from build123d import *

# Parameters (mm, degrees)
F0_W      = 127
F0_H      = 127
F1_DEPTH  = 127
F2_R      = 12.7
F3_DEPTH  = 6.35
F4_R      = 12.7
F5_DEPTH  = 6.35
F6_R      = 12.7
F7_DEPTH  = 6.35
F8_R      = 12.7
F9_DEPTH  = 6.35
F10_R     = 12.7
F11_DEPTH = 6.35
F12_R     = 12.7
F13_DEPTH = 6.35
F14_R     = 12.7
F15_DEPTH = 6.35
F16_R     = 12.7
F17_DEPTH = 6.35
F18_R     = 12.7
F19_DEPTH = 6.35
F20_R     = 12.2418661496
F21_DEPTH = 6.35
F22_R     = 12.7
F23_DEPTH = 6.35
F25_R     = 12.7
F26_DEPTH = 6.35
F27_R     = 12.7
F28_DEPTH = 6.35
F29_R     = 12.7
F30_DEPTH = 6.35
F31_R     = 12.7
F32_DEPTH = 6.35
F33_R     = 12.7
F34_DEPTH = 6.35
F35_R     = 12.7
F36_DEPTH = 6.35
F37_R     = 12.7
F38_DEPTH = 6.35
F39_R     = 12.7
F40_DEPTH = 6.35
F41_R     = 12.7
F42_DEPTH = 6.35
F43_R     = 12.7
F44_DEPTH = 6.35


# Not quite as in the source:
# - a length typed as a fraction of an inch, garbled in the dataset ("3 / 203.2 mm" for 3/8 in), is restored


with BuildPart() as f1:
    # F0 (on Right) → F1 (new body)
    with BuildSketch(Plane.YZ):
        with Locations((-2.1555427632, -5.2600353956)):
            Rectangle(F0_W, F0_H)
    extrude(amount=F1_DEPTH)

    # F2 (on face) → F3 (cut)
    with BuildSketch(Plane(origin=(0, 61.3444572368, 0), x_dir=(-1, 0, 0), z_dir=(0, 1, 0))):
        with Locations((-63.2817981055, -5.2596604964)):
            Circle(F2_R)
    extrude(amount=-F3_DEPTH, mode=Mode.SUBTRACT)

    # F4 (on face) → F5 (cut)
    with BuildSketch(Plane(origin=(0, 0, 0), x_dir=(0, -1, 0), z_dir=(-1, 0, 0))):
        with Locations((2.032, -6.35)):
            Circle(F4_R)
    extrude(amount=-F5_DEPTH, mode=Mode.SUBTRACT)

    # F6 (on face) → F7 (cut)
    with BuildSketch(Plane(origin=(0, 0, 0), x_dir=(0, -1, 0), z_dir=(-1, 0, 0))):
        with Locations((-39.1194572368, 36.0149646044)):
            Circle(F6_R)
    extrude(amount=-F7_DEPTH, mode=Mode.SUBTRACT)

    # F8 (on face) → F9 (cut)
    with BuildSketch(Plane(origin=(0, 0, 0), x_dir=(0, -1, 0), z_dir=(-1, 0, 0))):
        with Locations((43.4305427632, 36.0149646044)):
            Circle(F8_R)
    extrude(amount=-F9_DEPTH, mode=Mode.SUBTRACT)

    # F10 (on face) → F11 (cut)
    with BuildSketch(Plane(origin=(0, 0, 0), x_dir=(0, -1, 0), z_dir=(-1, 0, 0))):
        with Locations((-39.1194572368, -46.5350353956)):
            Circle(F10_R)
    extrude(amount=-F11_DEPTH, mode=Mode.SUBTRACT)

    # F12 (on face) → F13 (cut)
    with BuildSketch(Plane(origin=(0, 0, 0), x_dir=(0, -1, 0), z_dir=(-1, 0, 0))):
        with Locations((43.4305427632, -46.5350353956)):
            Circle(F12_R)
    extrude(amount=-F13_DEPTH, mode=Mode.SUBTRACT)

    # F14 (on face) → F15 (cut)
    with BuildSketch(Plane.YZ.offset(127)):
        with Locations((39.1194572368, -46.5350353956)):
            Circle(F14_R)
    extrude(amount=-F15_DEPTH, mode=Mode.SUBTRACT)

    # F16 (on face) → F17 (cut)
    with BuildSketch(Plane.YZ.offset(127)):
        with Locations((-43.4305427632, 36.0149646044)):
            Circle(F16_R)
    extrude(amount=-F17_DEPTH, mode=Mode.SUBTRACT)

    # F18 (on face) → F19 (cut)
    with BuildSketch(Plane.XZ.offset(65.6555427632)):
        with Locations((104.775, -46.5350353956)):
            Circle(F18_R)
    extrude(amount=-F19_DEPTH, mode=Mode.SUBTRACT)

    # F20 (on face) → F21 (cut)
    with BuildSketch(Plane.XZ.offset(65.6555427632)):
        with Locations((63.5, -46.5350353956)):
            Circle(F20_R)
    extrude(amount=-F21_DEPTH, mode=Mode.SUBTRACT)

    # F22 (on face) → F23 (cut)
    with BuildSketch(Plane.XZ.offset(65.6555427632)):
        with Locations((22.225, -46.5350353956)):
            Circle(F22_R)
    extrude(amount=-F23_DEPTH, mode=Mode.SUBTRACT)

    # F25 (on face) → F26 (cut)
    with BuildSketch(Plane.XZ.offset(65.6555427632)):
        with Locations((104.775, 36.0149646044)):
            Circle(F25_R)
    extrude(amount=-F26_DEPTH, mode=Mode.SUBTRACT)

    # F27 (on face) → F28 (cut)
    with BuildSketch(Plane.XZ.offset(65.6555427632)):
        with Locations((63.5, 36.0149646044)):
            Circle(F27_R)
    extrude(amount=-F28_DEPTH, mode=Mode.SUBTRACT)

    # F29 (on face) → F30 (cut)
    with BuildSketch(Plane.XZ.offset(65.6555427632)):
        with Locations((22.225, 36.0149646044)):
            Circle(F29_R)
    extrude(amount=-F30_DEPTH, mode=Mode.SUBTRACT)

    # F31 (on face) → F32 (cut)
    with BuildSketch(Plane.XY.offset(58.2399646044)):
        with Locations((104.775, -43.4305427632)):
            Circle(F31_R)
    extrude(amount=-F32_DEPTH, mode=Mode.SUBTRACT)

    # F33 (on face) → F34 (cut)
    with BuildSketch(Plane.XY.offset(58.2399646044)):
        with Locations((63.5, -2.1555427632)):
            Circle(F33_R)
    extrude(amount=-F34_DEPTH, mode=Mode.SUBTRACT)

    # F35 (on face) → F36 (cut)
    with BuildSketch(Plane.XY.offset(58.2399646044)):
        with Locations((22.225, 39.1194572368)):
            Circle(F35_R)
    extrude(amount=-F36_DEPTH, mode=Mode.SUBTRACT)

    # F37 (on face) → F38 (cut)
    with BuildSketch(Plane(origin=(0, 0, -68.7600353956), x_dir=(1, 0, 0), z_dir=(0, 0, -1))):
        with Locations((104.775, 43.4305427632)):
            Circle(F37_R)
    extrude(amount=-F38_DEPTH, mode=Mode.SUBTRACT)

    # F39 (on face) → F40 (cut)
    with BuildSketch(Plane(origin=(0, 0, -68.7600353956), x_dir=(1, 0, 0), z_dir=(0, 0, -1))):
        with Locations((22.225, 43.4305427632)):
            Circle(F39_R)
    extrude(amount=-F40_DEPTH, mode=Mode.SUBTRACT)

    # F41 (on face) → F42 (cut)
    with BuildSketch(Plane(origin=(0, 0, -68.7600353956), x_dir=(1, 0, 0), z_dir=(0, 0, -1))):
        with Locations((22.225, -39.1194572368)):
            Circle(F41_R)
    extrude(amount=-F42_DEPTH, mode=Mode.SUBTRACT)

    # F43 (on face) → F44 (cut)
    with BuildSketch(Plane(origin=(0, 0, -68.7600353956), x_dir=(1, 0, 0), z_dir=(0, 0, -1))):
        with Locations((104.775, -39.1194572368)):
            Circle(F43_R)
    extrude(amount=-F44_DEPTH, mode=Mode.SUBTRACT)


solid = f1.part
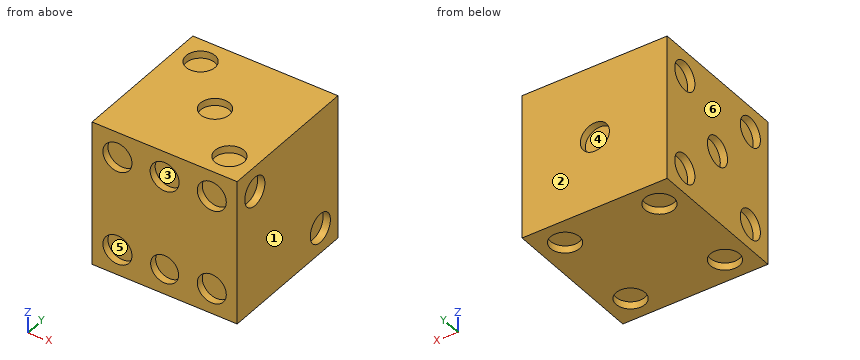
Work out the finished part from the listing and answer in its coordinate system (mm). Face numbers are marked on the shaded views. A direction names the side the tool comes from. Give positions to 0.01 mm unless a question says otherwise; leave off trailing zeros. Loops run counter-clockwise (first coordinate to the right, second up) from the corner with the lowest first, then second, coordinate; pieces in that order, holes last. Notation, with made-up numbers: (86.25, 12) - (111.25, 12) arc R36 cw to (111.25, 49) - close; hole circle Ø9 at (75.5, 37.25). An arc over 180 degrees is marked (long way). Answer in a Markdown table with one row per item. Add a question column.
Q1. Each of these flat-tipped pins is pushed along its axis until it touches: P1, Ø12.5, axis at y = -42.5, z = -49, coming from the -X side; P2, Ø12, axis at x = 29, z = 28.5, coming from the -Y side; P3, Ø12.5, axis at y = 36, z = -51, coming from the +X side; P4, Ø8, axis at x = 101.5, y = -49.5, coming from the +Z side. Where does it stop, or does it pass through?
Q2. The part is cut by section A-A (x = 102.5). Determine the outline of the cut face in (y, z), and give its area (3 significant figures).
Q3. Consider line 1 along Y through (x, z) = (3, -6); line 2 along Z through (x, y) = (19, -52.5); line 3 along Z through (x, y) = (5.5, 36). Determine where each line is inside the solid, lowest interval first.
Q4. The part is cut by section B-B (y = -49). Determine the outline of the cut face in (x, z).
Q5. Determine the mould class of the marked faces 1, 2 and 3 for opening direction X: released by +X, released by -X, zero draft, split by the parting line, or undercut.
Q6. The part is cut by section D-D (x = 63.5). Determine the outline of the cut face in (y, z), and give its area (3 significant figures).
Q7. A tool of negligible diameter and unlimited length cuts with its end or side. For the marked faces 4, 5 and 6, from which of +Z, -Z, +X, -X, +Y, -Y can it reach the whole face along a straight path? Write none if from no direction.
Q8. The part is cut by section C-C (z = -56). Determine the outline of the cut face in (x, y).
Solution:
| question | item | result |
|---|---|---|
| 1 | P1 | stops at x = 6.35 |
| 1 | P2 | stops at y = -65.66 |
| 1 | P3 | stops at x = 120.65 |
| 1 | P4 | stops at z = 51.89 |
| 2 | outline | (-65.66, -68.76) - (-55.93, -68.76) - (-55.93, -62.41) - (-30.94, -62.41) - (-30.94, -68.76) - (26.62, -68.76) - (26.62, -62.41) - (51.61, -62.41) - (51.61, -68.76) - (61.34, -68.76) - (61.34, 58.24) - (-30.94, 58.24) - (-30.94, 51.89) - (-55.93, 51.89) - (-55.93, 58.24) - (-65.66, 58.24) - (-65.66, 48.51) - (-59.31, 48.51) - (-59.31, 23.52) - (-65.66, 23.52) - (-65.66, -34.04) - (-59.31, -34.04) - (-59.31, -59.03) - (-65.66, -59.03) - close |
| 2 | area | 15,300 mm² |
| 3 | line 1 | y = -65.66 to -14.73, 10.66 to 61.34 |
| 3 | line 2 | z = -62.41 to 58.24 |
| 3 | line 3 | z = -68.76 to -58.85, -34.22 to 23.7, 48.33 to 58.24 |
| 4 | outline | (0, -68.76) - (10.81, -68.76) - (10.81, -62.41) - (33.64, -62.41) - (33.64, -68.76) - (93.36, -68.76) - (93.36, -62.41) - (116.19, -62.41) - (116.19, -68.76) - (127, -68.76) - (127, 24.6) - (120.65, 24.6) - (120.65, 47.43) - (127, 47.43) - (127, 58.24) - (116.19, 58.24) - (116.19, 51.89) - (93.36, 51.89) - (93.36, 58.24) - (0, 58.24) - (0, 47.43) - (6.35, 47.43) - (6.35, 24.6) - (0, 24.6) - (0, -35.12) - (6.35, -35.12) - (6.35, -57.95) - (0, -57.95) - close |
| 5 | face 1 | released by +X |
| 5 | face 2 | zero draft |
| 5 | face 3 | undercut |
| 6 | outline | (-65.66, -68.76) - (61.34, -68.76) - (61.34, -17.96) - (54.99, -17.96) - (54.99, 7.44) - (61.34, 7.44) - (61.34, 58.24) - (10.54, 58.24) - (10.54, 51.89) - (-14.86, 51.89) - (-14.86, 58.24) - (-65.66, 58.24) - (-65.66, 48.71) - (-59.31, 48.71) - (-59.31, 23.31) - (-65.66, 23.31) - (-65.66, -34.29) - (-59.31, -34.29) - (-59.31, -58.78) - (-65.66, -58.78) - close |
| 6 | area | 15,500 mm² |
| 7 | face 4 | +Y |
| 7 | face 5 | -Y |
| 7 | face 6 | +Z, -Z, -X, +Y, -Y |
| 8 | outline | (0, -65.66) - (13.76, -65.66) - (13.76, -59.31) - (30.69, -59.31) - (30.69, -65.66) - (55.74, -65.66) - (55.74, -59.31) - (71.26, -59.31) - (71.26, -65.66) - (96.31, -65.66) - (96.31, -59.31) - (113.24, -59.31) - (113.24, -65.66) - (127, -65.66) - (127, 30.65) - (120.65, 30.65) - (120.65, 47.59) - (127, 47.59) - (127, 61.34) - (0, 61.34) - (0, 47.59) - (6.35, 47.59) - (6.35, 30.65) - (0, 30.65) - (0, -34.96) - (6.35, -34.96) - (6.35, -51.9) - (0, -51.9) - close |
